For this review, take the finished solid that the model builds, in its own axes (mm). Face numbers are marked on the shaded views. A direction names the side the tool comes from. Give positions to 0.01 mm unless a question says otherwise; leave off trailing zeros. Write each loop counter-clockwise with the first axis right and the second up, starting at its lowest first coordinate (ties: lowest second). Pieces come first, ordered by that corner, then holes.
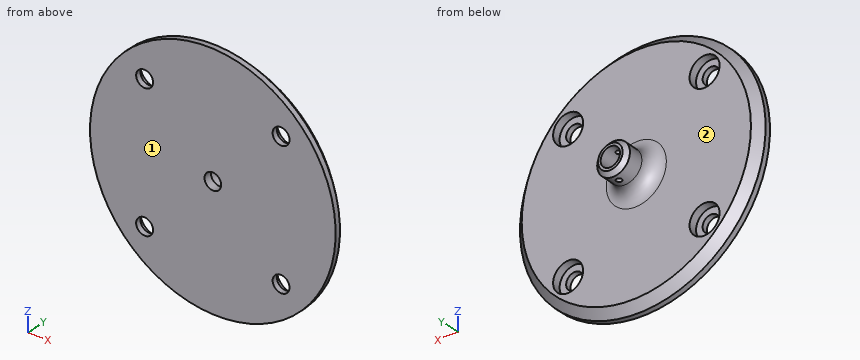
from build123d import *

# Parameters (mm, degrees)
SKETCH1_R               = 45
BOSS_EXTRUDE1_DEPTH     = 5
SKETCH2_R               = 3.1
CUT_EXTRUDE1_DEPTH      = 64.835726674
SKETCH8_R               = 5.5
CUT_EXTRUDE6_DEPTH      = 3
CIRPATTERN1_COUNT       = 4
SKETCH3_R               = 6
BOSS_EXTRUDE2_DEPTH     = 12
SKETCH4_R               = 3.55
CUT_EXTRUDE2_DEPTH      = 14
SKETCH5_R               = 3.05
CUT_EXTRUDE3_DEPTH      = 66.161338231
FILLET1_R               = 5
CUT_EXTRUDE5_DEPTH      = 66.871086221
CUT_EXTRUDE5_DEPTH_BACK = 66.871086221
SKETCH7_R               = 1
CHAMFER1_SIZE           = 3
CHAMFER2_SIZE           = 1.5


with BuildPart() as part:
    # Sketch1 → Boss-Extrude1 (new body)
    with BuildSketch(Plane(origin=(0, 0, 0), x_dir=(1, 0, 0), z_dir=(0, 1, 0))):
        with Locations(Location((0, 0, 0), (0, 0, 270))):
            Circle(SKETCH1_R)
    extrude(amount=BOSS_EXTRUDE1_DEPTH)

    # Sketch2 → Cut-Extrude1 (cut, through all)
    with BuildSketch(Plane(origin=(0, 5, 0), x_dir=(1, 0, 0), z_dir=(0, 1, 0))):
        with Locations(Location((-25, 25, 0), (0, 0, 270))):
            Circle(SKETCH2_R)
    cut_extrude1 = extrude(amount=-CUT_EXTRUDE1_DEPTH, mode=Mode.SUBTRACT)

    # Sketch8 → Cut-Extrude6 (cut)
    with BuildSketch(Plane(origin=(0, 5, 0), x_dir=(1, 0, 0), z_dir=(0, 1, 0))):
        with Locations(Location((-25, 25, 0), (0, 0, 270))):
            Circle(SKETCH8_R)
    cut_extrude6 = extrude(amount=-CUT_EXTRUDE6_DEPTH, mode=Mode.SUBTRACT)

    # CirPattern1: Cut-Extrude1, Cut-Extrude6 ×4 about axis
    cirpattern1_axis = Axis((0, 0, 0), (0, 1, 0))
    add([cut_extrude1.rotate(cirpattern1_axis, i * 360 / CIRPATTERN1_COUNT) for i in range(1, CIRPATTERN1_COUNT)], mode=Mode.SUBTRACT)
    add([cut_extrude6.rotate(cirpattern1_axis, i * 360 / CIRPATTERN1_COUNT) for i in range(1, CIRPATTERN1_COUNT)], mode=Mode.SUBTRACT)

    # Sketch3 → Boss-Extrude2 (add)
    with BuildSketch(Plane(origin=(0, 5, 0), x_dir=(1, 0, 0), z_dir=(0, 1, 0))):
        with Locations(Location((0, 0, 0), (0, 0, 270))):
            Circle(SKETCH3_R)
    extrude(amount=BOSS_EXTRUDE2_DEPTH)

    # Sketch4 → Cut-Extrude2 (cut)
    with BuildSketch(Plane(origin=(0, 17, 0), x_dir=(1, 0, 0), z_dir=(0, 1, 0))):
        with Locations(Location((0, 0, 0), (0, 0, 270))):
            Circle(SKETCH4_R)
    extrude(amount=-CUT_EXTRUDE2_DEPTH, mode=Mode.SUBTRACT)

    # Sketch5 → Cut-Extrude3 (cut, through all)
    with BuildSketch(Plane(origin=(0, 3, 0), x_dir=(1, 0, 0), z_dir=(0, 1, 0))):
        with Locations(Location((0, 0, 0), (0, 0, 270))):
            Circle(SKETCH5_R)
    extrude(amount=-CUT_EXTRUDE3_DEPTH, mode=Mode.SUBTRACT)

    # Fillet1
    fillet1_edges = [part.edges().sort_by_distance(p)[0] for p in [
        (0, 5, -6),
    ]]
    fillet(fillet1_edges, radius=FILLET1_R)

    # Sketch7 → Cut-Extrude5 (cut, two sides: drawn at the far end of the back side and taken through both)
    with BuildSketch(Plane(origin=(0, 0, 0), x_dir=(-1, 0, 0), z_dir=(0, 0, -1)).offset(-CUT_EXTRUDE5_DEPTH_BACK)):
        with Locations((0, 13)):
            Circle(SKETCH7_R)
    extrude(amount=CUT_EXTRUDE5_DEPTH + CUT_EXTRUDE5_DEPTH_BACK, mode=Mode.SUBTRACT)

    # Chamfer1
    chamfer1_edges = [part.edges().sort_by_distance(p)[0] for p in [
        (0, 5, -45),
    ]]
    chamfer(chamfer1_edges, length=CHAMFER1_SIZE)

    # Chamfer2
    chamfer2_edges = [part.edges().sort_by_distance(p)[0] for p in [
        (0, 17, -6),
    ]]
    chamfer(chamfer2_edges, length=CHAMFER2_SIZE)


solid = part.part
(1) We need section C-C (y = 7.75). Write out the cut boundary in (x, z), and give its area (3 significant figures).
(2) We need section A-A (z = 0). Write out the cut boundary in (x, y), and give its area (3 significant figures).
(3) Tool access review of the marked faces 1 and 2: name each direction out of +Z, -Z, +X, -X, +Y, -Y from which nothing blocks a thin tool from reaching the whole face with its end or side.
(4) Clearance check with flat-ended pins moving along their axes: pin 1 Ø9 at (x, z) = (-27, 25) entering from +Y; pin 2 Ø6.5 at (x, z) = (-25, 25) entering from +Y; pin 3 Ø4 at (y, z) = (3, 29) entering from -X. State where each tip first meets the part, or that it passes through.
(5) We need section B-B (x = 25). Count the separate pieces of the cut face and the enclosed holes in it, and give its area (3 significant figures).
(6) For L1, parallel to Z at x = -29, y = 4; L2, parallel to X at y = 11.25, z = 0; L3, parallel to Y at x = 38, z = -2, list the stretches that pass through material, from the lowest coordinate up.
The answers:
1. outline: circle Ø13.07 at (0, 0); hole circle Ø7.1 at (0, 0)
1. area: 94.6 mm2
2. outline: (-45, 0) - (-3.05, 0) - (-3.05, 3) - (-3.55, 3) - (-3.55, 17) - (-4.5, 17) - (-6, 15.5) - (-6, 10) arc R5 cw to (-11, 5) - (-42, 5) - (-45, 2) - close; (3.05, 0) - (45, 0) - (45, 2) - (42, 5) - (11, 5) arc R5 cw to (6, 10) - (6, 15.5) - (4.5, 17) - (3.55, 17) - (3.55, 3) - (3.05, 3) - close
2. area: 476 mm2
3. face 1: +Z, -Z, +X, -X, -Y
3. face 2: +Y
4. pin 1: stops at y = 5
4. pin 2: stops at y = 2
4. pin 3: stops at x = -35.8
5. separate pieces: 3
5. enclosed holes: 0
5. area: 272 mm2
6. L1: z = -31.75 to -28.77, -21.23 to 21.23, 28.77 to 31.75
6. L2: x = -6 to -3.55, 3.55 to 6
6. L3: y = 0 to 5
